For this review, use the dimensioned drawing (mm, ordinates from the lowest corner) and the shaded views. Round coordinates to 2 decimals unless told otherwise and drop trailing zeros. Loops run counter-clockwise (first coordinate to the right, second up) from the corner with the lowest first, then second, coordinate; pieces in that order, holes last. Notation, with made-up numbers: M 2.5,-36 L 36.5,-36 A21 ccw 36.5,-20 Z; hole C 64,77 d4. An arc over 180 degrees is marked long. One line per item, written item: value. Start each with the question number.
Item 1: We need section B-B (y = 4). Write out the cut boundary in (x, z).
Item 2: Clearance check with a flat-ended pin moving along its axis: pin 1 (2.5 mm diameter, centred on x = 4, y = 4, fed in from -Z). State where the tip first meets the part, or that it passes through.
Item 3: For line 1 along Y through (x, z) = (141, 1.2); line 2 along X through (y, z) = (76, 1.2), list the stretches that pass through material, from the lowest coordinate up.
Item 4: We need section A-A (x = 4). Write out the cut boundary in (y, z), then the cut area to 3 significant figures.
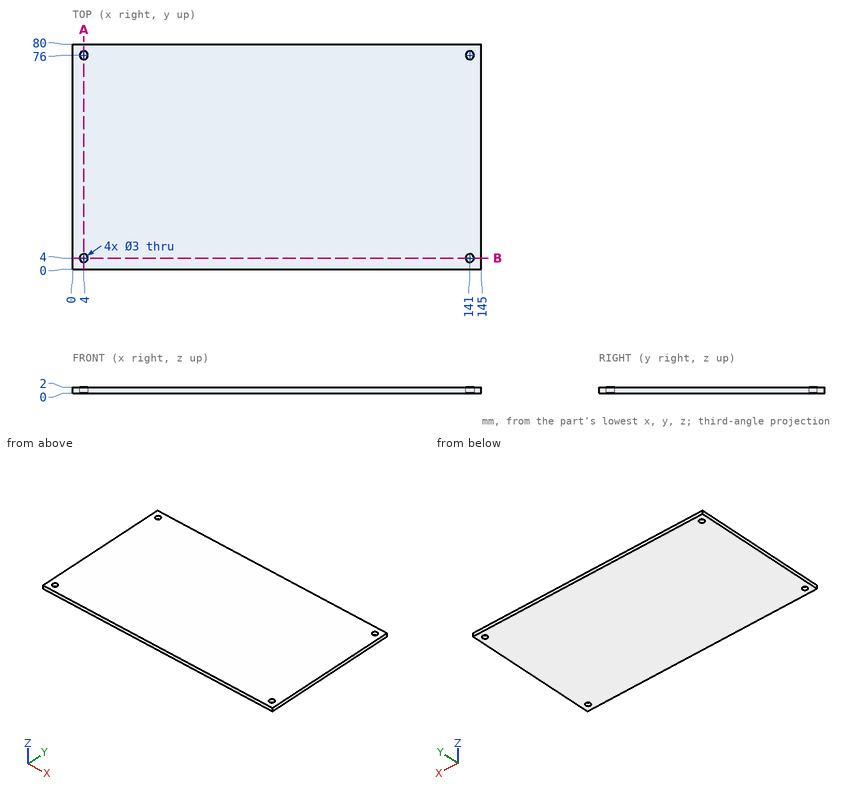
A:
1. outline: M 0,0 L 2.5,0 L 2.5,2 L 0,2 Z; M 5.5,0 L 139.5,0 L 139.5,2 L 5.5,2 Z; M 142.5,0 L 145,0 L 145,2 L 142.5,2 Z
2. pin 1: through
3. line 1: 0 to 2.5, 5.5 to 74.5, 77.5 to 80
3. line 2: 0 to 2.5, 5.5 to 139.5, 142.5 to 145
4. outline: M 0,0 L 2.5,0 L 2.5,2 L 0,2 Z; M 5.5,0 L 74.5,0 L 74.5,2 L 5.5,2 Z; M 77.5,0 L 80,0 L 80,2 L 77.5,2 Z
4. area: 148 mm2
